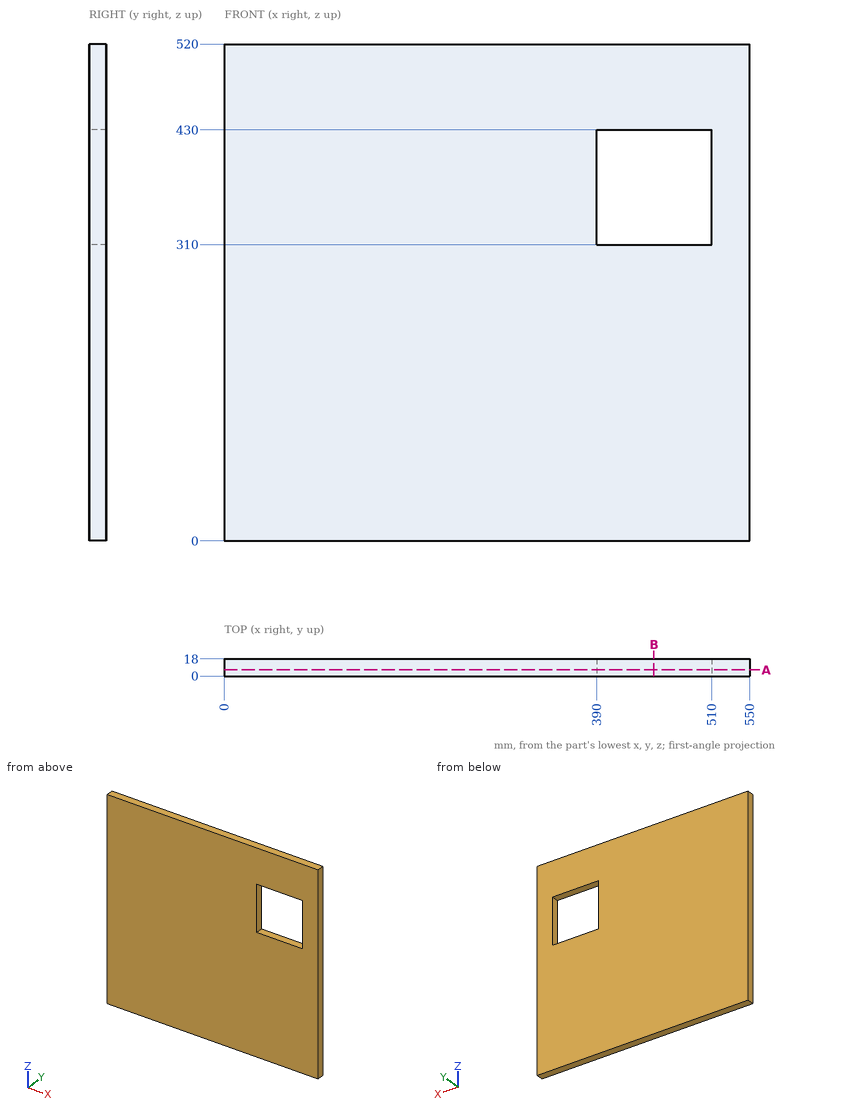
Source: three-view drawing plus pictorial views. Frame: mm from the lowest corner of the part. Coordinates: 2 decimals unless noted, no trailing zeros. Write each loop counter-clockwise with the first axis right and the second up, starting at its lowest first coordinate (ties: lowest second). Pieces come first, ordered by that corner, then holes. Notation, with made-up numbers: (34, 41) -> (77, 41) arc R25 cw to (77, 78) -> close; hole circle Ø8 at (-16.5, 36.5). An arc over 180 degrees is marked (long way). Answer as a JSON object with one key per item and string values.
1. Section A-A on y = 6.5. Return the cut outline in (x, z).
Result set:
{"outline": "(0, 0) -> (550, 0) -> (550, 520) -> (0, 520) -> close; hole (390, 310) -> (510, 310) -> (510, 430) -> (390, 430) -> close"}
2. Section B-B on x = 449.5. Return the cut outline in (y, z), then the cut area to 3 significant figures.
Result set:
{"outline": "(0, 0) -> (18, 0) -> (18, 310) -> (0, 310) -> close; (0, 430) -> (18, 430) -> (18, 520) -> (0, 520) -> close", "area": "7,200 mm2"}
3. Material intervals for line 1 (X direction, y = 12.5, z = 349); line 2 (Z direction, x = 485, y = 13.5), sorted ascending. Write a range as from..to.
Result set:
{"line 1": "x = 0..390, 510..550", "line 2": "z = 0..310, 430..520"}
